The listing builds one solid part. Answer for the finished solid, in the listing's coordinates (mm). Face numbers are marked on the shaded views. A direction names the side the tool comes from. Coordinates: 2 decimals unless noted, no trailing zeros. Loops run counter-clockwise (first coordinate to the right, second up) from the corner with the lowest first, then second, coordinate; pieces in that order, holes last. Notation, with made-up numbers: (67.25, 78) - (112.25, 78) arc R29 cw to (112.25, 102) - close; hole circle Ø8 at (-37, 36). An arc over 180 degrees is marked (long way). Write each question's results on one line, items separated by ' | '. Start each with the question number.
(1) Find section D-D on z = 26.5. Determine the outline of the cut face in (x, y).
(2) Find section C-C on x = 15. Determine the outline of the cut face in (y, z), then the cut area to 3 significant figures.
(3) Consider line 1 (Z direction, x = 280, y = 144.5); line 2 (X direction, y = -3, z = 15); line 3 (X direction, y = 143, z = 95). Determine where each line is inside the solid, lowest interval first. Write a range as from..to.
(4) Find section A-A on x = 185. Determine the outline of the cut face in (y, z), then the cut area to 3 significant figures.
(5) Find section B-B on y = 131. Determine the outline of the cut face in (x, z).
(6) For the marked faces 1, 2, 3 and 4, determine the directions among +Z, -Z, +X, -X, +Y, -Y from which every point of the face is accessible in a straight line to the end or side of a thin tool.
(7) Given pin 1 Ø10.5 at (x, z) = (14.5, 96) entering from +Y; pin 2 Ø4 at (y, z) = (94, 27) entering from +X; pin 3 Ø8 at (y, z) = (35, 28) entering from -X; pin 4 Ø17 at (x, z) = (185, 95) entering from -Y, each flat-ended and moving along its own axis, determine where each tip first touches the part or whether it passes through.
(8) Determine the mould class of the marked faces 5, 6, 7 and 8 for opening direction Y: released by +Y, released by -Y, zero draft, split by the parting line, or undercut.
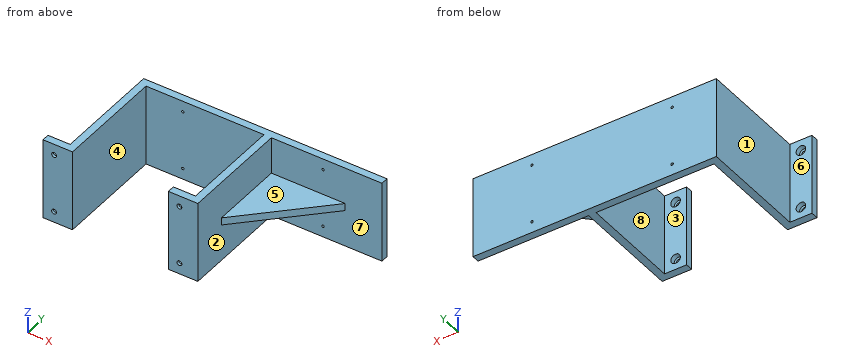
from build123d import *

# Parameters (mm, degrees)
BOSS_EXTRUDE1_DEPTH = 110
SKETCH2_R           = 3.3
CUT_EXTRUDE1_DEPTH  = 11
SKETCH3_R           = 6.5
CUT_EXTRUDE2_DEPTH  = 6.6
SKETCH5_W           = 150
SKETCH5_H           = 10
BOSS_EXTRUDE2_DEPTH = 110
BOSS_EXTRUDE3_DEPTH = 5
M4_TAPPED_HOLE1_D   = 3.3


with BuildPart() as part:
    # Sketch1 → Boss-Extrude1 (new body)
    with BuildSketch(Plane.XY):
        Polygon((0, 0), (30, 0), (30, 147), (210, 147), (210, -10), (170, -10), (170, 0), (200, 0), (200, 137), (40, 137), (40, -10), (0, -10), align=None)
    extrude(amount=BOSS_EXTRUDE1_DEPTH)

    # Sketch2 → Cut-Extrude1 (cut, through all)
    with BuildSketch(Plane(origin=(0, 0, 0), x_dir=(1, 0, 0), z_dir=(0, 1, 0))):
        with Locations((15, -15)):
            Circle(SKETCH2_R)
        with Locations((15, -95)):
            Circle(SKETCH2_R)
        with Locations((185, -95)):
            Circle(SKETCH2_R)
        with Locations((185, -15)):
            Circle(SKETCH2_R)
    extrude(amount=-CUT_EXTRUDE1_DEPTH, mode=Mode.SUBTRACT)

    # Sketch3 → Cut-Extrude2 (cut)
    with BuildSketch(Plane(origin=(0, 0, 0), x_dir=(1, 0, 0), z_dir=(0, 1, 0))):
        with Locations((15, -15)):
            Circle(SKETCH3_R)
        with Locations((15, -95)):
            Circle(SKETCH3_R)
        with Locations((185, -95)):
            Circle(SKETCH3_R)
        with Locations((185, -15)):
            Circle(SKETCH3_R)
    extrude(amount=-CUT_EXTRUDE2_DEPTH, mode=Mode.SUBTRACT)

    # Sketch5 → Boss-Extrude2 (add)
    with BuildSketch(Plane.XY.offset(110)):
        with Locations((285, 142)):
            Rectangle(SKETCH5_W, SKETCH5_H)
    extrude(amount=-BOSS_EXTRUDE2_DEPTH)

    # Sketch6 → Boss-Extrude3 (add, symmetric)
    with BuildSketch(Plane.XY.offset(55)):
        Polygon((210, 37), (310, 137), (210, 137), align=None)
    extrude(amount=BOSS_EXTRUDE3_DEPTH, both=True)

    # M4 Tapped Hole1 (through all)
    with Locations(Plane(origin=(0, 147, 0), x_dir=(1, 0, 0), z_dir=(0, 1, 0))):
        with Locations((90, -15), (280, -15), (280, -95), (90, -95)):
            Hole(M4_TAPPED_HOLE1_D / 2)


solid = part.part
Values:
1) outline: (0, -10) - (40, -10) - (40, 137) - (200, 137) - (200, 0) - (170, 0) - (170, -10) - (210, -10) - (210, 137) - (360, 137) - (360, 147) - (30, 147) - (30, 0) - (0, 0) - close
2) outline: (-10, 0) - (0, 0) - (0, 8.5) - (-6.6, 8.5) - (-6.6, 11.7) - (-10, 11.7) - close; (-10, 18.3) - (-6.6, 18.3) - (-6.6, 21.5) - (0, 21.5) - (0, 88.5) - (-6.6, 88.5) - (-6.6, 91.7) - (-10, 91.7) - close; (-10, 98.3) - (-6.6, 98.3) - (-6.6, 101.5) - (0, 101.5) - (0, 110) - (-10, 110) - close | area: 884 mm²
3) line 1: z = 0..13.35, 16.65..93.35, 96.65..110 | line 2: x = 0..8.5, 21.5..40, 170..178.5, 191.5..210 | line 3: x = 30..88.35, 91.65..278.35, 281.65..360
4) outline: (-10, 0) - (0, 0) - (0, 8.5) - (-6.6, 8.5) - (-6.6, 11.7) - (-10, 11.7) - close; (-10, 18.3) - (-6.6, 18.3) - (-6.6, 21.5) - (0, 21.5) - (0, 88.5) - (-6.6, 88.5) - (-6.6, 91.7) - (-10, 91.7) - close; (-10, 98.3) - (-6.6, 98.3) - (-6.6, 101.5) - (0, 101.5) - (0, 110) - (-10, 110) - close; (137, 0) - (147, 0) - (147, 110) - (137, 110) - close | area: 1,980 mm²
5) outline: (30, 0) - (40, 0) - (40, 110) - (30, 110) - close; (200, 0) - (210, 0) - (210, 50) - (304, 50) - (304, 60) - (210, 60) - (210, 110) - (200, 110) - close
6) face 1: +Z, -Z, -X, +Y | face 2: +X, -Y | face 3: +Z, -Z | face 4: +Z, -Z, -Y
7) pin 1: stops at y = -6.6 | pin 2: stops at x = 210 | pin 3: stops at x = 30 | pin 4: stops at y = -10
8) face 5: zero draft | face 6: released by +Y | face 7: released by -Y | face 8: undercut
